Can you work these out from the model? Positions are in its coordinate system, mm. A direction names the side the tool comes from. Coordinates: 2 decimals unless noted, no trailing zeros. Write each loop counter-clockwise with the first axis right and the second up, starting at its lowest first coordinate (ties: lowest second). Pieces come first, ordered by that corner, then holes. Notation, with made-up numbers: (26, -35) - (40, -35) arc R14 cw to (40, -14) - close; hole circle Ø4 at (76, -29). An arc over 180 degrees is marked (long way). Use one line per item in the form item = value. Start each with the question number.
(1) If we section it at A-A on y = 15: Please give me the cut outline in (x, z) (3 decimals).
(2) If we section it at B-B on z = -1.1: Please give me the cut outline in (x, y) (3 decimals), then the cut area to 3 significant figures.
(3) On a 3-axis mill with a long thin cutter (end or side, diameter ignored), from which of +Z, -Z, +X, -X, +Y, -Y can I reach the whole of each face in a straight line? I mean faces 1 (the face through (0.875, 12, 2)), 2 (the face through (-2, 12, 0.875)), 3 (the face through (-2, 12, -0.875)), 4 (the face through (-2.39, 12.26, -0.01)), 5 (the face through (2, 12, -0.875)). Say none if no direction works.
(4) For pin 1 Ø0.9 at (y, z) = (10.5, -1.5) entering from -X; pin 2 Ø0.7 at (y, z) = (16, 1.5) entering from -X; pin 3 Ø0.9 at (x, y) = (-2, 12.5) entering from -Z (3 decimals), each with a flat end and sliding along its axis, tell me the tip position at first contact or that it passes through.
(5) If we section it at C-C on x = -1.15: Please give me the cut outline in (y, z) (3 decimals), then the cut area to 3 significant figures.
(6) If I drill on probe 1 along X at (y, z) = (3.75, -1.55) (3 decimals); probe 2 along Z at (x, y) = (0.1, 7.5), over which ranges is the centre line in solid material (lowest first)? Write a range as from..to.
```python
from build123d import *

# Parameters (mm, degrees)
SKETCH1_W          = 2.39
SKETCH1_H          = 24.195
CUT_EXTRUDE1_DEPTH = 25.195
CUT_EXTRUDE2_DEPTH = 25.195
CUT_EXTRUDE3_DEPTH = 25.195
CUT_EXTRUDE4_DEPTH = 25.195
FILLET1_R          = 0.5


with BuildPart() as part:
    # Sketch1 → Revolve1 (revolve)
    with BuildSketch(Plane(origin=(0, 0, 0), x_dir=(-1, 0, 0), z_dir=(0, 0, -1))):
        with Locations((-1.195, 12.0975)):
            Rectangle(SKETCH1_W, SKETCH1_H)
    revolve(axis=Axis((0, 0, 0), (0, 1, 0)))

    # Sketch2 → Cut-Extrude1 (cut, through all)
    with BuildSketch(Plane.XZ):
        with BuildLine():
            Line((0.875, 2.22406722), (0.875, 0.875))
            Line((0.875, 0.875), (2.22406722, 0.875))
            ThreePointArc((2.22406722, 0.875), (1.689985207, 1.689985207), (0.875, 2.22406722))
        make_face()
    extrude(amount=-CUT_EXTRUDE1_DEPTH, mode=Mode.SUBTRACT)

    # Sketch3 → Cut-Extrude2 (cut, through all)
    with BuildSketch(Plane.XZ):
        with BuildLine():
            Line((2.22406722, -0.875), (0.875, -0.875))
            Line((0.875, -0.875), (0.875, -2.22406722))
            ThreePointArc((0.875, -2.22406722), (1.689985207, -1.689985207), (2.22406722, -0.875))
        make_face()
    extrude(amount=-CUT_EXTRUDE2_DEPTH, mode=Mode.SUBTRACT)

    # Sketch4 → Cut-Extrude3 (cut, through all)
    with BuildSketch(Plane.XZ):
        with BuildLine():
            Line((-0.875, -2.22406722), (-0.875, -0.875))
            Line((-0.875, -0.875), (-2.22406722, -0.875))
            ThreePointArc((-2.22406722, -0.875), (-1.689985207, -1.689985207), (-0.875, -2.22406722))
        make_face()
    extrude(amount=-CUT_EXTRUDE3_DEPTH, mode=Mode.SUBTRACT)

    # Sketch5 → Cut-Extrude4 (cut, through all)
    with BuildSketch(Plane.XZ):
        with BuildLine():
            Line((-2.22406722, 0.875), (-0.875, 0.875))
            Line((-0.875, 0.875), (-0.875, 2.22406722))
            ThreePointArc((-0.875, 2.22406722), (-1.689985207, 1.689985207), (-2.22406722, 0.875))
        make_face()
    extrude(amount=-CUT_EXTRUDE4_DEPTH, mode=Mode.SUBTRACT)

    # Fillet1
    fillet1_edges = [part.edges().sort_by_distance(p)[0] for p in [
        (2.39, 0, 0),
        (0.875, 12.0975, 0.875),
        (0, 24.195, -2.39),
        (0, 0, -2.39),
        (0.875, 12.0975, -0.875),
        (-2.39, 24.195, 0),
        (-2.39, 0, 0),
        (-0.875, 12.0975, -0.875),
        (0, 24.195, 2.39),
        (0, 0, 2.39),
        (-0.875, 12.0975, 0.875),
        (2.39, 24.195, 0),
    ]]
    fillet(fillet1_edges, radius=FILLET1_R)


solid = part.part
```
Reported:
q1.outline = (-2.224, -0.875) - (-1.375, -0.875) arc R0.5 cw to (-0.875, -1.375) - (-0.875, -2.224) arc R2.39 ccw to (0.875, -2.224) - (0.875, -1.375) arc R0.5 cw to (1.375, -0.875) - (2.224, -0.875) arc R2.39 ccw to (2.224, 0.875) - (1.375, 0.875) arc R0.5 cw to (0.875, 1.375) - (0.875, 2.224) arc R2.39 ccw to (-0.875, 2.224) - (-0.875, 1.375) arc R0.5 cw to (-1.375, 0.875) - (-2.224, 0.875) arc R2.39 ccw to start
q2.outline = (-0.957, 0) - (0.957, 0) - (0.957, 24.195) - (-0.957, 24.195) - close
q2.area = 46.3 mm2
q3.face_1 = +Z, +X, +Y, -Y
q3.face_2 = +Z, -X, +Y, -Y
q3.face_3 = -Z, -X, +Y, -Y
q3.face_4 = -X, +Y, -Y
q3.face_5 = -Z, +X, +Y, -Y
q4.pin_1 = -1
q4.pin_2 = -0.93
q4.pin_3 = -0.875
q5.outline = (0, -0.928) - (24.195, -0.928) - (24.195, 0.928) - (0, 0.928) - close
q5.area = 44.9 mm2
q6.probe_1 = -0.875..0.875
q6.probe_2 = -2.39..2.39
